Source: CAD feature listing. Evaluate the final solid. Frame: model axes, mm. A direction names the side the tool comes from. Round coordinates to 2 decimals unless told otherwise and drop trailing zeros. Order: outer loops, then holes, each group sorted by start corner. A loop starts at its lowest first (then second) coordinate and runs counter-clockwise, first axis right, second up. Notation, with made-up numbers: (59.25, -5.5) - (117.25, -5.5) arc R11 ccw to (117.25, 13.5) - close; hole circle Ø5 at (28, 48). An arc over 180 degrees is marked (long way). Return JSON: item names as keys, results as strings. Group by question number.
1) Access query for faces 5 (the cylindrical face through (0.098, 3.215, -1.699)), 6 (the cylindrical face through (0.098, 0.285, -1.699)), 7 (the cylindrical face through (6.79, 2.36, 0.99)). Directions: +Z, -Z, +X, -X, +Y, -Y. A direction counts if a zero-diameter tool reaches every point of the face in a straight line with its end or side. Return the directions, or none.
2) Contact query for flat-ended pins moving along their axis: P1, Ø1, axis at y = 0.5, z = -4.5, coming from the +X side; P2, Ø1.7, axis at x = -1.5, y = 1.5, coming from the -Z side; P3, Ø1.8, axis at y = 1.75, z = -6, coming from the +X side. Output: stop coordinate, or through.
3) Section D-D, the plane y = 2.3. Return loops of the section in (x, z), plus the area to 3 significant figures.
4) Section A-A, the plane z = -3.5. Return loops of the section in (x, y), plus the area to 3 significant figures.
5) Section B-B, the plane x = -6. Return loops of the section in (y, z), plus the area to 3 significant figures.
6) Section C-C, the plane z = -6. Return loops of the section in (x, y), plus the area to 3 significant figures.
7) Ray query, line 1 (Z direction, x = 9.3, y = 1.75); line 2 (X direction, y = 2.2, z = -3.25); line 3 (Y direction, x = -8.3, z = -6). Return the intervals inside material, ascending. Write a range as from..to.
8) Mould query, pull axis X, two halves, no side actions, for faces 1 (the cylindrical face through (0.217, 2.726, 0.986)), 2 (the cylindrical face through (-9.699, 0.285, -4.056)), 3 (the flat face through (0.1, 0.6, 0)), 4 (the flat face through (6, 2, 2)). Classes: pulls with the +X half, pulls with the -X half, needs draft (parallel to the pull), parting line crosses it, or undercut.
```python
from build123d import *

# Parameters (mm, degrees)
SALIENTE_EXTRUIR1_DEPTH = 3.5
CROQUIS2_R              = 1
SALIENTE_EXTRUIR2_DEPTH = 2
REDONDEO1_R             = 1
CROQUIS3_R              = 1
CORTAR_EXTRUIR1_DEPTH   = 20.111514854


with BuildPart() as part:
    # Croquis1 → Saliente-Extruir1 (new body)
    with BuildSketch(Plane(origin=(0, 0, 0), x_dir=(1, 0, 0), z_dir=(0, 1, 0))):
        Polygon((10, 0), (-10, 0), (-10, 8), (-7, 8), (-7, 2), (7, 2), (7, 8), (10, 8), align=None)
    extrude(amount=SALIENTE_EXTRUIR1_DEPTH)

    # Croquis2 → Saliente-Extruir2 (add)
    with BuildSketch(Plane.XY):
        with Locations(Location((0, 1.75, 0), (0, 0, 180))):
            Circle(CROQUIS2_R)
        with Locations(Location((-6, 1.75, 0), (0, 0, 180))):
            Circle(CROQUIS2_R)
        with Locations(Location((6, 1.75, 0), (0, 0, 180))):
            Circle(CROQUIS2_R)
    extrude(amount=SALIENTE_EXTRUIR2_DEPTH)

    # Redondeo1
    redondeo1_edges = [part.edges().sort_by_distance(p)[0] for p in [
        (0, 0, -2),
        (-10, 3.5, -4),
        (10, 3.5, -4),
        (0, 3.5, -2),
        (10, 0, -4),
        (-10, 0, -4),
    ]]
    fillet(redondeo1_edges, radius=REDONDEO1_R)

    # Croquis3 → Cortar-Extruir1 (cut, through all)
    with BuildSketch(Plane(origin=(-7, 0, 0), x_dir=(0, 0, -1), z_dir=(1, 0, 0))):
        with Locations((6, 1.75)):
            Circle(CROQUIS3_R)
    cortar_extruir1 = extrude(amount=-CORTAR_EXTRUIR1_DEPTH, mode=Mode.SUBTRACT)

    # Simetría3: Cortar-Extruir1 across plane
    add(cortar_extruir1.mirror(Plane(origin=(0, 0, 0), x_dir=(0, 0, 1), z_dir=(1, 0, 0))), mode=Mode.SUBTRACT)


solid = part.part
```
Geometry check:
{
 "1": {"face 5": "-Z, +Y", "face 6": "-Z, -Y", "face 7": "+Z"},
 "2": {"P1": "x = 10", "P2": "z = -2", "P3": "through"},
 "3": {"outline": "(-10, -8) - (-7, -8) - (-7, -6.84) - (-10, -6.84) - close; (-10, -5.16) - (-7, -5.16) - (-7, -2) - (7, -2) - (7, -5.16) - (10, -5.16) - (10, 0) - (6.84, 0) - (6.84, 2) - (5.16, 2) - (5.16, 0) - (0.84, 0) - (0.84, 2) - (-0.84, 2) - (-0.84, 0) - (-5.16, 0) - (-5.16, 2) - (-6.84, 2) - (-6.84, 0) - (-10, 0) - close; (7, -8) - (10, -8) - (10, -6.84) - (7, -6.84) - close", "area": "76.0 mm2"},
 "4": {"outline": "(-10, 1) arc R1 ccw to (-9, 0) - (-7, 0) - (-7, 3.5) - (-9, 3.5) arc R1 ccw to (-10, 2.5) - close; (7, 0) - (9, 0) arc R1 ccw to (10, 1) - (10, 2.5) arc R1 ccw to (9, 3.5) - (7, 3.5) - close", "area": "20.1 mm2"},
 "5": {"outline": "(0, -1) arc R1 ccw to (1, -2) - (2.5, -2) arc R1 ccw to (3.5, -1) - (3.5, 0) - (2.75, 0) - (2.75, 2) - (0.75, 2) - (0.75, 0) - (0, 0) - close", "area": "10.6 mm2"},
 "6": {"outline": "(-9.97, 0.75) arc R1 ccw to (-9, 0) - (-7, 0) - (-7, 0.75) - close; (-9.97, 2.75) - (-7, 2.75) - (-7, 3.5) - (-9, 3.5) arc R1 ccw to start; (7, 0) - (9, 0) arc R1 ccw to (9.97, 0.75) - (7, 0.75) - close; (7, 2.75) - (9.97, 2.75) arc R1 ccw to (9, 3.5) - (7, 3.5) - close", "area": "8.15 mm2"},
 "7": {"line 1": "-8..-7, -5..0", "line 2": "-10..-7, 7..10", "line 3": "0..0.75, 2.75..3.5"},
 "8": {"face 1": "undercut", "face 2": "pulls with the -X half", "face 3": "undercut", "face 4": "needs draft"}
}
